Autodesk Inventor part; units mm, degrees
ref_plane "YZ Plane" through (0, 0, 0) normal (1, 0, 0) x (0, 1, 0)
ref_plane "XZ Plane" through (0, 0, 0) normal (0, 1, 0) x (-1, 0, 0)
ref_plane "XY Plane" through (0, 0, 0) normal (0, 0, 1) x (1, 0, 0)
sketch "Sketch1" plane through (0, 0, 0) normal (1, 0, 0) x (0, 1, 0)
  line L0 (0, 0) -> (-25.4, 0)
  line L1 (-25.4, 0) -> (-25.4, -25.4)
  line L2 (-25.4, -25.4) -> (0, -25.4)
  line L3 (0, -25.4) -> (0, 0)
  dimension "d0" = 25.4
  dimension "d1" = 25.4
extrude "Extrusion1" add sketch "Sketch1" along normal blind 406.4
sketch "Sketch2" plane through (406.4, 0, 0) normal (1, 0, 0) x (0, 0, -1)
  circle A0 centre (12.7, -12.7) radius 6.35
  line L0 (12.7, -12.7) -> (12.7, 0) construction
  line L1 (25.4, 0) -> (0, 0)
  dimension "d4" = 12.7
  dimension "d11" = 12.7
extrude "Extrusion2" add sketch "Sketch2" along normal blind 18.796
sketch "Sketch3" plane through (0, 0, 0) normal (-1, 0, 0) x (0, 0, 1)
  circle A0 centre (-12.7, -12.7) radius 6.35
  line L0 (-12.7, -12.7) -> (-12.7, 0) construction
  line L1 (-25.4, 0) -> (0, 0) construction
  line L2 (0, 0) -> (0, -25.4) construction
  dimension "d9" = 12.7
  dimension "d10" = 12.7
extrude "Extrusion3" add sketch "Sketch3" against normal blind 19.05
sketch "Sketch4" plane through (0, -25.4, 0) normal (0, 0, 1) x (1, 0, 0)
  line L0 (0, 25.4) -> (403.86, 25.4)
  line L1 (403.86, 25.4) -> (403.86, 30.48)
  line L2 (403.86, 30.48) -> (0, 30.48)
  line L3 (0, 30.48) -> (0, 25.4)
  dimension "d12" = 5.08
  dimension "d15" = 403.86
extrude "Extrusion4" add sketch "Sketch4" against normal blind 177.8
properties part number "hopper_bar"
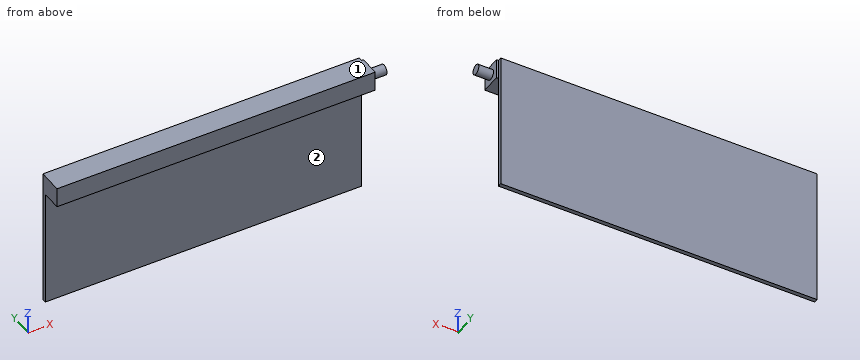
Check sheet for the modelled part. Datum: model origin and axes. Units: mm. Face numbers are marked on the shaded views. A direction names the side the tool comes from. Round coordinates to 2 decimals unless told otherwise and drop trailing zeros. Write each loop counter-clockwise with the first axis right and the second up, starting at its lowest first coordinate (ties: lowest second). Pieces come first, ordered by that corner, then holes. Notation, with made-up numbers: (-15, 78.5) -> (21, 78.5) arc R22 cw to (21, 102.5) -> close; hole circle Ø1 at (-38.75, 5). An arc over 180 degrees is marked (long way). Answer as CSV lines item,"result". Start each with the question number.
1) Tool access check on the marked faces 1 and 2. Record the directions out of +Z, -Z, +X, -X, +Y, -Y that give a thin tool (end or side, any length) a straight path to the whole face; none if there is none.
2) Section check D-D on z = -46. Enter the section's corners in (x, y).
3) Go/stop test with flat-tipped pins: P1, Ø6, axis at y = -2, z = -49.5, coming from the +X side; P2, Ø2, axis at x = 405.5, z = -11, coming from the +Y side; P3, Ø5, axis at x = 352, y = -6.5, coming from the -Z side. Record where each tip stops, or that it passes through.
4) Material ranges on line 1 (Y direction, x = 301.5, z = -83.5); line 2 (Z direction, x = 86.5, y = -1); line 3 (X direction, y = -2.5, z = -16.5), recorded low to high. Write a range as from..to.
5) Section check A-A on y = -12.7. Enter the section's corners in (x, z).
6) Section check B-B on z = -12.7. Enter the section's corners in (x, y), and give its area (3 significant figures).
7) Section check C-C on x = 152.5. Enter the section's corners in (y, z).
Found:
1,face 1,"+Z, +X, -X, +Y, -Y"
1,face 2,"-Z, +X, -X, -Y"
2,outline,"(0, 0) -> (403.86, 0) -> (403.86, 5.08) -> (0, 5.08) -> close"
3,P1,"stops at x = 403.86"
3,P2,"stops at y = 0"
3,P3,"stops at z = -25.4"
4,line 1,"y = 0..5.08"
4,line 2,"z = -25.4..0"
4,line 3,"x = 0..406.4"
5,outline,"(0, -25.4) -> (406.4, -25.4) -> (406.4, -19.05) -> (425.2, -19.05) -> (425.2, -6.35) -> (406.4, -6.35) -> (406.4, 0) -> (0, 0) -> close"
6,outline,"(0, -25.4) -> (406.4, -25.4) -> (406.4, -19.05) -> (425.2, -19.05) -> (425.2, -6.35) -> (406.4, -6.35) -> (406.4, 0) -> (403.86, 0) -> (403.86, 5.08) -> (0, 5.08) -> close"
6,area,"12,600 mm^2"
7,outline,"(-25.4, -25.4) -> (0, -25.4) -> (0, -177.8) -> (5.08, -177.8) -> (5.08, 0) -> (-25.4, 0) -> close"
